Work out the finished part from the listing and answer in its coordinate system (mm). A direction names the side the tool comes from. Round coordinates to 2 decimals unless told otherwise and drop trailing zeros. Order: outer loops, then holes, each group sorted by start corner. A loop starts at its lowest first (then second) coordinate and runs counter-clockwise, first axis right, second up. Notation, with made-up numbers: (33, -14) -> (42, -14) arc R15 cw to (42, -2) -> close; hole circle Ø1 at (56, -38.5). An arc over 180 degrees is marked (long way). Use one line per item in the form item = value.
```python
from build123d import *

# Parameters (mm, degrees)
SKETCH1_R           = 3.25
BOSS_EXTRUDE1_DEPTH = 17.686
SKETCH3_W           = 12.2
SKETCH3_H           = 6.9
BOSS_EXTRUDE2_DEPTH = 10
FILLET1_R           = 2.54
FILLET2_R           = 0.75
SKETCH5_W           = 2.032
SKETCH5_H           = 2.032
BOSS_EXTRUDE3_DEPTH = 2


with BuildPart() as part:
    # Sketch1 → Boss-Extrude1 (new body)
    with BuildSketch(Plane(origin=(0, 0, 0), x_dir=(1, 0, 0), z_dir=(0, 1, 0))):
        Circle(SKETCH1_R)
    extrude(amount=BOSS_EXTRUDE1_DEPTH)

    # Sketch3 → Boss-Extrude2 (add)
    with BuildSketch(Plane(origin=(0, 17.686, 0), x_dir=(1, 0, 0), z_dir=(0, 1, 0))):
        Rectangle(SKETCH3_W, SKETCH3_H)
    extrude(amount=BOSS_EXTRUDE2_DEPTH)

    # Fillet1
    fillet1_edges = [part.edges().sort_by_distance(p)[0] for p in [
        (6.1, 22.686, 3.45),
        (6.1, 22.686, -3.45),
        (-6.1, 22.686, -3.45),
        (-6.1, 22.686, 3.45),
    ]]
    fillet(fillet1_edges, radius=FILLET1_R)

    # Fillet2
    fillet2_edges = [part.edges().sort_by_distance(p)[0] for p in [
        (-6.1, 27.686, 0),
        (0, 27.686, -3.45),
        (6.1, 27.686, 0),
        (0, 27.686, 3.45),
        (-5.356051224, 27.686, 2.706051224),
        (5.356051224, 27.686, 2.706051224),
        (5.356051224, 27.686, -2.706051224),
        (-5.356051224, 27.686, -2.706051224),
    ]]
    fillet(fillet2_edges, radius=FILLET2_R)

    # Sketch5 → Boss-Extrude3 (add)
    with BuildSketch(Plane.XZ.offset(-17.686)):
        with Locations((-2.286, -4.466)):
            Rectangle(SKETCH5_W, SKETCH5_H)
        with Locations((1.651, 4.466)):
            Rectangle(SKETCH5_W, SKETCH5_H)
    extrude(amount=-BOSS_EXTRUDE3_DEPTH)


solid = part.part
```
Item 1: The part is cut by section C-C, the plane z = 0. Give the vertices of the cut face in (x, y).
Findings:
outline = (-6.1, 17.69) -> (-3.25, 17.69) -> (-3.25, 0) -> (3.25, 0) -> (3.25, 17.69) -> (6.1, 17.69) -> (6.1, 26.94) arc R0.75 ccw to (5.35, 27.69) -> (-5.35, 27.69) arc R0.75 ccw to (-6.1, 26.94) -> close
Item 2: The part is cut by section A-A, the plane y = 20.25. Give the vertices of the cut face in (x, z), and give its area (3 significant figures).
Findings:
outline = (-6.1, -0.91) arc R2.54 ccw to (-3.56, -3.45) -> (3.56, -3.45) arc R2.54 ccw to (6.1, -0.91) -> (6.1, 0.91) arc R2.54 ccw to (3.56, 3.45) -> (-3.56, 3.45) arc R2.54 ccw to (-6.1, 0.91) -> close
area = 78.6 mm^2
Item 3: The part is cut by section B-B, the plane x = 0. Give the vertices of the cut face in (y, z), and give its area (3 significant figures).
Findings:
outline = (0, -3.25) -> (17.69, -3.25) -> (17.69, -3.45) -> (26.94, -3.45) arc R0.75 ccw to (27.69, -2.7) -> (27.69, 2.7) arc R0.75 ccw to (26.94, 3.45) -> (17.69, 3.45) -> (17.69, 3.25) -> (0, 3.25) -> close
area = 184 mm^2
Item 4: The part is cut by section D-D, the plane x = -2.75. Give the vertices of the cut face in (y, z), and give its area (3 significant figures).
Findings:
outline = (0, -1.73) -> (17.69, -1.73) -> (17.69, -5.48) -> (19.69, -5.48) -> (19.69, -3.45) -> (26.94, -3.45) arc R0.75 ccw to (27.69, -2.7) -> (27.69, 2.7) arc R0.75 ccw to (26.94, 3.45) -> (17.69, 3.45) -> (17.69, 1.73) -> (0, 1.73) -> close
area = 134 mm^2
Item 5: Flat-ended cylindrical pins translate along their axes: P1, Ø1.6, axis at x = 2, z = 4, coming from the +Y side (3 decimals); P2, Ø0.6, axis at y = 19, z = -4.5, coming from the -X side; P3, Ø1.6, axis at y = 18, z = -4, coming from the +X side. Find the tip coordinate at first contact, or state that the pin passes through.
Findings:
P1 = 27.495
P2 = -3.3
P3 = 4.66
Item 6: Consider line 1 along Z through (x, y) = (2, 18); line 2 along Y through (x, z) = (-4.5, 2); line 3 along X through (y, z) = (1.5, 0). Determine where each line is inside the solid, lowest interval first.
Findings:
line_1 = -3.45 to 5.48
line_2 = 17.69 to 27.69
line_3 = -3.25 to 3.25
Item 7: For faces 1 (the flat face through (-3, 17.686, 2)), 2 (the flat face through (2.667, 19, 4)), 3 (the flat face through (-1.27, 19, -4)), 4 (the flat face through (-2, 19.686, -4)), determine the directions among +Z, -Z, +X, -X, +Y, -Y from which every point of the face is accessible in a straight line to the end or side of a thin tool.
Findings:
face_1 = -Y
face_2 = +Z, +X, +Y, -Y
face_3 = -Z, +X, +Y, -Y
face_4 = -Z, +X, -X, +Y
